from build123d import *

# Parameters (mm, degrees)
BOSS_EXTRUDE1_DEPTH   = 30
BODY_MOVE_COPY1_ANGLE = 60
SCALE1_SCALE_X        = 1
SCALE1_SCALE_Y        = 1
SCALE1_SCALE_Z        = 1.1
CIRPATTERN2_COUNT     = 3
BOSS_EXTRUDE3_DEPTH   = 30


with BuildPart() as part:
    # Sketch1 → Boss-Extrude1 (new body)
    with BuildSketch(Plane.XY):
        Polygon((200, -115.470053838), (200, 115.470053838), (100, 57.735026919), (100, -57.735026919), align=None)
    extrude(amount=BOSS_EXTRUDE1_DEPTH)


with BuildPart() as body_2:
    # Body-Move_Copy1: copy of part
    add(part.part.rotate(Axis((0, 0, 0), (0, 0, 1)), BODY_MOVE_COPY1_ANGLE))


with BuildPart() as body_2_1:
    # Scale1: scaled about (77.777777778, 134.715062811, 15)
    add(body_2.part.scale((SCALE1_SCALE_X, SCALE1_SCALE_Y, SCALE1_SCALE_Z), about=(77.777777778, 134.715062811, 15)))

    # Combine1: union part
    add(part.part)


with BuildPart() as cirpattern2_1:
    # CirPattern2: pattern copy
    add(body_2_1.part.rotate(Axis((0, 0, 0), (0, 0, 1)), 1 * 360 / CIRPATTERN2_COUNT))


with BuildPart() as cirpattern2_2:
    # CirPattern2: pattern copy
    add(body_2_1.part.rotate(Axis((0, 0, 0), (0, 0, 1)), 2 * 360 / CIRPATTERN2_COUNT))


with BuildPart() as body_2_2:
    add(body_2_1.part)

    add(cirpattern2_1.part)  # Boss-Extrude3 merges CirPattern2_1

    add(cirpattern2_2.part)  # Boss-Extrude3 merges CirPattern2_2
    # Sketch2 → Boss-Extrude3 (add)
    with BuildSketch(Plane(origin=(0, 0, 0), x_dir=(-1, 0, 0), z_dir=(0, 0, -1))):
        Polygon((-200, 115.470053838), (0, 230.940107676), (200, 115.470053838), (200, -115.470053838), (0, -230.940107676), (-200, -115.470053838), align=None)
    extrude(amount=BOSS_EXTRUDE3_DEPTH)


solid = body_2_2.part
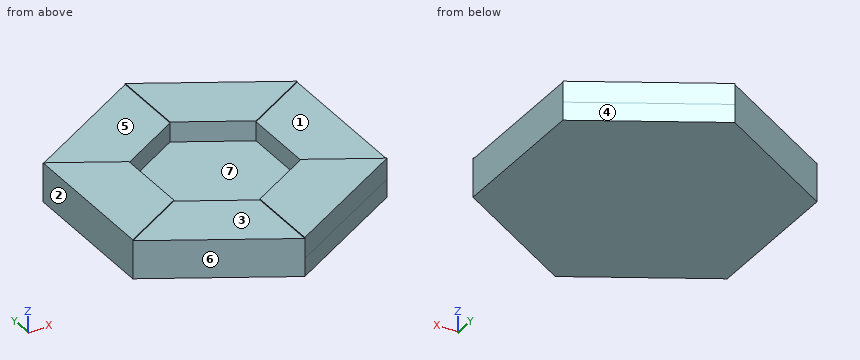
Can you work these out from the model? Positions are in its coordinate system, mm. Face numbers are marked on the shaded views. A direction names the side the tool comes from. Give positions to 0.01 mm unless a question says otherwise; leave off trailing zeros. Loops run counter-clockwise (first coordinate to the right, second up) from the corner with the lowest first, then second, coordinate; pieces in that order, holes last. Notation, with made-up numbers: (-34.5, 41) -> (0.5, 41) arc R20 ccw to (0.5, 46) -> close; hole circle Ø7 at (-8, -37.75). An arc over 180 degrees is marked (long way). Write item = value, one per line.
1) I need wall thicknesses on L1, parallel to Z at x = -157, y = -98.5; L2, parallel to X at y = 2, z = 0.5; L3, parallel to Y at x = 86.5, z = 25.5. Which ranges of each line are inside material? Lowest first, please. Write a range as from..to.
Check result:
L1 = -30..30
L2 = -200..-100, 100..200
L3 = -181..-65.53, 65.53..181
2) Will these pins go through, and if not, where does the flat tip stop? pin 1 (1 mm diameter, centred on x = 58.5, z = -2, fed in from +Y); pin 2 (6 mm diameter, centred on y = -146.5, z = -10.5, fed in from -X); pin 3 (5 mm diameter, centred on y = -144.5, z = 18, fed in from -X).
Check result:
pin_1 = 197.45
pin_2 = -151.45
pin_3 = -154.05
3) Suppose I cut it at B-B on x = -73.5. Write out the boundary of the cut face in (y, z).
Check result:
outline = (-188.5, -30) -> (188.5, -30) -> (188.5, 30) -> (73.03, 30) -> (73.03, 0) -> (-73.03, 0) -> (-73.03, 30) -> (-188.5, 30) -> close
4) Thinking about a two-plate mould opening in X: for the marked faces 4, 5, 6 and 7, which applies, released by +X, released by -X, zero draft, split by the parting line, or undercut?
Check result:
face_4 = released by +X
face_5 = undercut
face_6 = released by -X
face_7 = undercut
5) Suppose I cut it at A-A on z = -23. Write out the boundary of the cut face in (x, y), then the cut area to 3 significant figures.
Check result:
outline = (-200, -115.47) -> (0, -230.94) -> (200, -115.47) -> (200, 115.47) -> (0, 230.94) -> (-200, 115.47) -> close
area = 139,000 mm2
6) For the marked faces 1, 2 and 3, which set-ups out of +Z, -Z, +X, -X, +Y, -Y let a thin tool reach every point of the face, with its end or its side?
Check result:
face_1 = +Z, +X
face_2 = +Z, -Z, -X, +Y, -Y
face_3 = +Z, -Y
